from build123d import *

# Parameters (mm, degrees)
EXTRUDE_1_DEPTH      = 10
EXTRUDE_1_DEPTH_BACK = 10
EXTRUDE_START        = -30
SKETCH_2_R           = 30
EXTRUDE_2_DEPTH      = 30


with BuildPart() as part:
    # 草图1 → 凸台-拉伸1 (new, two sides: drawn at the far end of the back side and taken through both)
    with BuildSketch(Plane.XY.offset(-EXTRUDE_1_DEPTH_BACK)):
        with BuildLine():
            Line((159.099025767, 30), (-159.099025767, 30))
            ThreePointArc((-159.099025767, 30), (-189.099025767, 0), (-159.099025767, -30))
            Line((-159.099025767, -30), (159.099025767, -30))
            ThreePointArc((159.099025767, -30), (189.099025767, 0), (159.099025767, 30))
        make_face()
    extrude(amount=EXTRUDE_1_DEPTH + EXTRUDE_1_DEPTH_BACK)

    # 草图2 → 凸台-拉伸2 (add)
    with BuildSketch(Plane.XY.offset(EXTRUDE_START)):
        with Locations((-159.099025767, 0)):
            Circle(SKETCH_2_R)
    extrude(amount=EXTRUDE_2_DEPTH)


solid = part.part
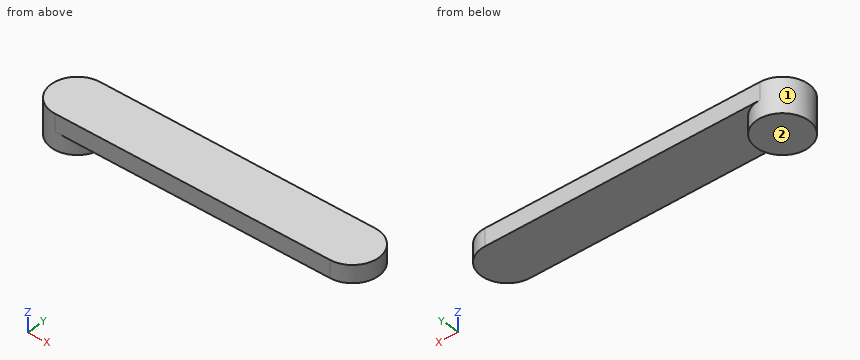
Geometry check sheet. Reference: the model listing, model coordinates, mm. Face numbers are marked on the shaded views. A direction names the side the tool comes from. Give positions to 0.01 mm unless a question says otherwise; leave off trailing zeros. Write each loop counter-clockwise with the first axis right and the second up, starting at its lowest first coordinate (ties: lowest second). Pieces come first, ordered by that corner, then holes. Notation, with made-up numbers: (16, -27.5) - (63, -27.5) arc R21 cw to (63, -12.5) - close; hole circle Ø5 at (61.5, -26.5). An arc over 180 degrees is marked (long way). Put each result on its own line as item: value.
1. Thickness scan on line 1 (Z direction, x = -81, y = -23); line 2 (X direction, y = -11.5, z = -27.5); line 3 (X direction, y = 23, z = 5). Record the ranges inside material, lowest first.
Ans:
line 1: z = -10 to 10
line 2: x = -186.81 to -131.39
line 3: x = -178.36 to 178.36
2. Sectioned sample at B-B, the plane z = 4. Enter the section's corners in (x, y).
Ans:
outline: (-159.1, -30) - (159.1, -30) arc R30 ccw to (159.1, 30) - (-159.1, 30) arc R30 ccw to start
3. Sectioned sample at D-D, the plane y = -18. Enter the section's corners in (x, z).
Ans:
outline: (-183.1, -30) - (-135.1, -30) - (-135.1, -10) - (183.1, -10) - (183.1, 10) - (-183.1, 10) - close
4. Sectioned sample at A-A, the plane y = 0. Enter the section's corners in (x, z), plus the area to 3 significant figures.
Ans:
outline: (-189.1, -30) - (-129.1, -30) - (-129.1, -10) - (189.1, -10) - (189.1, 10) - (-189.1, 10) - close
area: 8,760 mm²
5. Go/stop test with flat-tipped pins: pin 1 (8 mm diameter, centred on y = -19, z = -1, fed in from +X); pin 2 (1 mm diameter, centred on y = 6.5, z = -11, fed in from +X); pin 3 (5 mm diameter, centred on y = 16.5, z = -15.5, fed in from -X). Record where each tip stops, or that it passes through.
Ans:
pin 1: stops at x = 185.08
pin 2: stops at x = -129.71
pin 3: stops at x = -185.63
6. Sectioned sample at C-C, the plane x = -147.5. Enter the section's corners in (y, z), plus the area to 3 significant figures.
Ans:
outline: (-30, -10) - (-27.67, -10) - (-27.67, -30) - (27.67, -30) - (27.67, -10) - (30, -10) - (30, 10) - (-30, 10) - close
area: 2,310 mm²
7. Set-up check for the marked faces 1 and 2: record each of +Z, -Z, +X, -X, +Y, -Y from which the full face is reachable in a straight line by a thin tool's end or side.
Ans:
face 1: -Z
face 2: -Z, +X, -X, +Y, -Y
